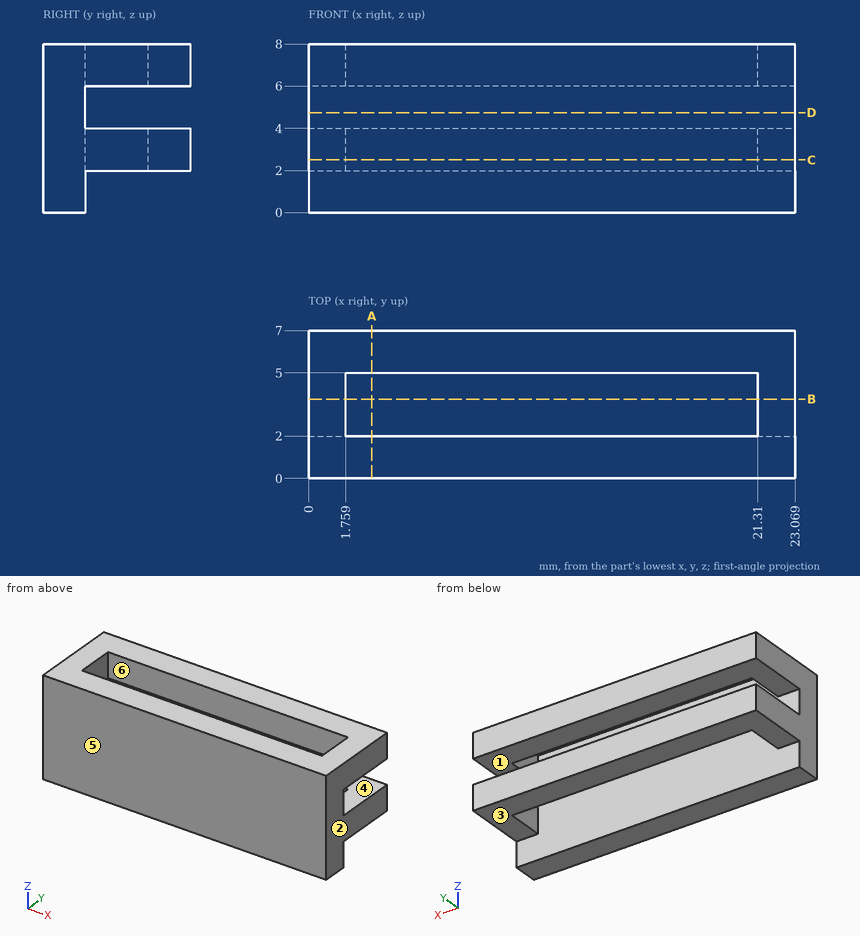
The drawing under review shows one solid part. Ordinate dimensions are in mm from its lowest x, y, z. A direction names the side the tool comes from. Give positions to 0.01 mm unless a question says otherwise; leave off trailing zeros. Write each loop counter-clockwise with the first axis right and the second up, starting at its lowest first coordinate (ties: lowest second). Pieces come first, ordered by that corner, then holes. Notation, with made-up numbers: (35.25, -28.5) - (84.25, -28.5) arc R20 cw to (84.25, -2.5) - close; hole circle Ø2 at (-9, -8.5). An arc over 180 degrees is marked (long way). Answer in a Markdown table with one row per item. Add a question column.
1. Tool access review of the marked faces 5 and 6: name each direction out of +Z, -Z, +X, -X, +Y, -Y from which nothing blocks a thin tool from reaching the whole face with its end or side.
2. Draft analysis for pull direction Z (two halves, no side actions). For the marked faces 1, 2, 3 and 4, state which applies: +Z half, -Z half, draft (parallel to the pull), parting line (faces both ways), or undercut.
3. We need section D-D on z = 4.75. Write out the cut boundary in (x, y).
4. Insertion check: P1, Ø1.5, axis at x = 9.5, y = 5.5, coming from the -Z side. The pin has a flat end and moves straight along its axis. Give the tip position at first contact, or say it passes through.
5. We need section C-C on z = 2.5. Write out the cut boundary in (x, y), then the cut area to 3 significant figures.
6. Wall thickness on line 1 along Z through (x, y) = (22.25, 5.75); line 2 along Y through (x, z) = (14.5, 3.5); line 3 along X through (y, z) = (3, 7): over which ranges is each line inside the solid? List them lowest first. Write a range as [from, to].
7. We need section A-A on x = 3. Write out the cut boundary in (y, z).
8. We need section B-B on y = 3.75. Write out the cut boundary in (x, z).
Ans:
| question | item | result |
|---|---|---|
| 1 | face 5 | +Z, -Z, +X, -X, -Y |
| 1 | face 6 | +Z, -Z |
| 2 | face 1 | undercut |
| 2 | face 2 | draft |
| 2 | face 3 | -Z half |
| 2 | face 4 | undercut |
| 3 | outline | (0, 0) - (23.07, 0) - (23.07, 2) - (0, 2) - close |
| 4 | P1 | stops at z = 2 |
| 5 | outline | (0, 0) - (23.07, 0) - (23.07, 7) - (0, 7) - close; hole (1.76, 2) - (21.31, 2) - (21.31, 5) - (1.76, 5) - close |
| 5 | area | 103 mm^2 |
| 6 | line 1 | z = [2, 4], [6, 8] |
| 6 | line 2 | y = [0, 2], [5, 7] |
| 6 | line 3 | x = [0, 1.76], [21.31, 23.07] |
| 7 | outline | (0, 0) - (2, 0) - (2, 8) - (0, 8) - close; (5, 2) - (7, 2) - (7, 4) - (5, 4) - close; (5, 6) - (7, 6) - (7, 8) - (5, 8) - close |
| 8 | outline | (0, 2) - (1.76, 2) - (1.76, 4) - (0, 4) - close; (0, 6) - (1.76, 6) - (1.76, 8) - (0, 8) - close; (21.31, 2) - (23.07, 2) - (23.07, 4) - (21.31, 4) - close; (21.31, 6) - (23.07, 6) - (23.07, 8) - (21.31, 8) - close |
